```python
from build123d import *

# Parameters (mm, degrees)
BOSS_EXTRUDE1_DEPTH = 10
SKETCH2_R           = 3.175
CUT_EXTRUDE1_DEPTH  = 86.380649173
SKETCH3_R           = 5
CUT_EXTRUDE2_DEPTH  = 80.450837411
FILLET1_R           = 10


with BuildPart() as part:
    # Sketch1 → Boss-Extrude1 (new, symmetric)
    with BuildSketch(Plane.XY):
        Polygon((-10, 70), (10, 70), (53.121778265, 47.990381057), (68.121778265, 22.009618943), (63.791651246, 19.509618943), (49.028935235, 45.079393131), (10, 65), (-10, 65), align=None)
    extrude(amount=BOSS_EXTRUDE1_DEPTH, both=True)

    # Sketch2 → Cut-Extrude1 (cut, through all)
    with BuildSketch(Plane(origin=(0, 70, 0), x_dir=(1, 0, 0), z_dir=(0, 1, 0))):
        with Locations(Location((0, 0, 0), (0, 0, 270))):
            Circle(SKETCH2_R)
    extrude(amount=-CUT_EXTRUDE1_DEPTH, mode=Mode.SUBTRACT)

    # Sketch3 → Cut-Extrude2 (cut, through all)
    with BuildSketch(Plane(origin=(60.621778265, 35, 0), x_dir=(0, 0, -1), z_dir=(0.8660254037844397, 0.499999999999998, 0))):
        with Locations(Location((0, 0, 0), (0, 0, 90))):
            Circle(SKETCH3_R)
    extrude(amount=-CUT_EXTRUDE2_DEPTH, mode=Mode.SUBTRACT)

    # Fillet1
    fillet1_edges = [part.edges().sort_by_distance(p)[0] for p in [
        (65.956714755, 20.759618943, -10),
        (65.956714755, 20.759618943, 10),
        (-10, 67.5, -10),
        (-10, 67.5, 10),
    ]]
    fillet(fillet1_edges, radius=FILLET1_R - 0.0001)  # a hair under: the kernel refuses the full size


solid = part.part
```
Build history of the part. All positions in model axes, mm. A direction names the side the tool comes from. Coordinates: 2 decimals unless noted, no trailing zeros. Order: outer loops, then holes, each group sorted by start corner. A loop starts at its lowest first (then second) coordinate and runs counter-clockwise, first axis right, second up. Notation, with made-up numbers: M 28,-16.75 L 47,-16.75 A28 cw 47,2.25 Z; hole C 55,-24.75 d10. An arc over 180 degrees is marked long. One line per question, with ' | ' between items. Start each with the question number.
1. Mould opens along X. For faces 3 (the face through (-1.93, 67.54, -2.52)), 4 (the face through (64.423, 23.346, 7.148)), 5 (the face through (-7.15, 67.54, 6.99)) say: +X half, -X half, draft (parallel to the pull), parting line (faces both ways), or undercut.
2. Wall check: line 1 along Y through (x, z) = (5.5, -8); line 2 along X through (y, z) = (67.05, 0) (3 decimals); line 3 along X through (y, z) = (66.5, 0) (3 decimals). Give the ranges that are in metal, low to high. Write a range as [from, to].
3. Tool access for faces 1 (the face through (2.4, 65, 2.4)), 2 (the face through (64.423, 23.346, -7.148)): list every direction of +Z, -Z, +X, -X, +Y, -Y with a clear straight run to the whole face (end or side of a thin tool).
4. Cut at C-C (y = 41.5). Write the cut outline in (x, z).
5. Flat gauge pins, fed straight in: P1, Ø1, axis at x = 45, z = -4.5, coming from the -Y side; P2, Ø6, axis at x = 53, z = -6, coming from the -Y side; P3, Ø5, axis at x = 32, z = -2, coming from the +Y side; P4, Ø1.5, axis at x = 55, y = 32.5, coming from the -Z side. Where does each tip first touch, or does it go through?
6. Cut at B-B (x = 6). Write the cut outline in (y, z).
7. Cut at A-A (z = -8.25). Write the cut outline in (x, y), plus the area to 3 significant figures.
The answers:
1) face 3: undercut | face 4: +X half | face 5: -X half
2) line 1: y = [65, 70] | line 2: x = [-10, -3.175], [3.175, 15.78] | line 3: x = [-10, -3.175], [3.175, 16.857]
3) face 1: +Z, -Z, -X, -Y | face 2: -Z, +X, -Y
4) outline: M 51.1,-10 L 56.87,-10 L 56.87,10 L 51.1,10 Z
5) P1: stops at y = 46.88 | P2: stops at y = 33.01 | P3: stops at y = 60.05 | P4: passes through
6) outline: M 65,-10 L 70,-10 L 70,10 L 65,10 Z
7) outline: M -5.65,65 L 10,65 L 49.03,45.08 L 61.62,23.28 L 65.95,25.78 L 53.12,47.99 L 10,70 L -5.65,70 Z | area: 411 mm2
